```python
from build123d import *

# Parameters (mm, degrees)
F1_DEPTH = 3.048
F2_COUNT = 10


with BuildPart() as f1:
    # F0 (on Top) → F1 (new body)
    with BuildSketch(Plane.XY):
        with BuildLine():
            ThreePointArc((0, 8.598116), (-0.985363, 8.91828), (-1.594351, 9.75648))
            ThreePointArc((-1.594351, 9.75648), (-2.322928, 11.1463), (-3.470461, 12.216624))
            ThreePointArc((-3.470461, 12.216624), (-3.924516, 12.078418), (-4.373089, 11.923342))
            ThreePointArc((-4.373089, 11.923342), (-4.672342, 10.382929), (-4.444858, 8.830294))
            ThreePointArc((-4.444858, 8.830294), (-4.444858, 7.794222), (-5.053846, 6.956022))
            Line((-5.053846, 6.956022), (0, 0))
            Line((0, 0), (0, 8.598116))
        make_face()
    extrude(amount=F1_DEPTH)

    # F2: F1 ×10 about axis
    f2_axis = Axis((0, 0, 1.524), (0, 0, 1))


with BuildPart() as f1_1:
    add(f1.part)
    for i in range(1, F2_COUNT):
        add(f1.part.rotate(f2_axis, i * 360 / F2_COUNT))


solid = f1_1.part
```
Geometry: final body of the model. Coordinates: model frame, mm. A direction names the side the tool comes from. Coordinates: 2 decimals unless noted, no trailing zeros. Write each loop counter-clockwise with the first axis right and the second up, starting at its lowest first coordinate (ties: lowest second). Pieces come first, ordered by that corner, then holes. Notation, with made-up numbers: M 0.25,-26.75 L 38.25,-26.75 A20 cw 38.25,3.25 Z; hole C 12,3.5 d2. An arc over 180 degrees is marked long. Answer as CSV lines item,"result". Start each with the question number.
Q1. Mould query, pull axis X, two halves, no side actions, for faces 4 (the cylindrical face through (12.7, 0, 1.5)), 5 (the cylindrical face through (-2.336, -11.164, 1.503)), 6 (the cylindrical face through (-11.339, -1.228, 1.503)), 7 (the cylindrical face through (8.41, -7.646, 1.503)). Classes: released by +X, released by -X, zero draft, split by the parting line, or undercut.
Q2. Pin query (flat end, axial travel): P1, Ø1.5, axis at y = 6, z = 2.5, coming from the -X side. Return the tip coordinate at first contact, or that it passes through.
Q3. Cut plane A-A on x = 1.25. Return the cut outline in (y, z).
Q4. Cut plane B-B on y = 5.25. Return the cut outline in (x, z), then the cut area to 3 significant figures.
Q5. Line query: line 1 (Y direction, x = 9, z = 2.15); line 2 (Y direction, x = -9.25, z = 2.45); line 3 (X direction, y = 7, z = 2.75). Output: solid intervals per line, ascending. Write a range as from..to.
Q6. Reachability of faces 1 (the cylindrical face through (2.31, -11.13, 1.5)), 2 (the cylindrical face through (-8.41, 7.646, 1.503)), 3 (the cylindrical face through (-9.895, 5.672, 1.503)) from +Z, -Z, +X, -X, +Y, -Y: full face, straight path, thin tool, end or side. Return the list, or none.
Findings below:
1,face 4,"released by +X"
1,face 5,"undercut"
1,face 6,"released by -X"
1,face 7,"undercut"
2,P1,"stops at x = -10.44"
3,outline,"M -9.16,0 L 9.16,0 L 9.16,3.05 L -9.16,3.05 Z"
4,outline,"M -9.57,0 L 9.57,0 L 9.57,3.05 L -9.57,3.05 Z"
4,area,"58.3 mm2"
5,line 1,"y = -7.78..-4.7, -1.69..1.69, 4.7..7.78"
5,line 2,"y = -7.82..-4.92, -1.58..1.58, 4.92..7.82"
5,line 3,"x = -10.52..-7.09, -5..5, 7.09..10.52"
6,face 1,"+Z, -Z, -Y"
6,face 2,"+Z, -Z, +Y"
6,face 3,"+Z, -Z, -X"
